Job drawing, mm, ordinate dimensions from the low corner. One solid piece. A direction names the side the tool comes from. Coordinates: 2 decimals unless noted, no trailing zeros. Loops run counter-clockwise (first coordinate to the right, second up) from the corner with the lowest first, then second, coordinate; pieces in that order, holes last. Notation, with made-up numbers: (14, -3.75) -> (71, -3.75) arc R11 cw to (71, 13.25) -> close; hole circle Ø3 at (42.5, 49). An arc over 180 degrees is marked (long way). Answer as CSV lines item,"result". Start each with the question number.
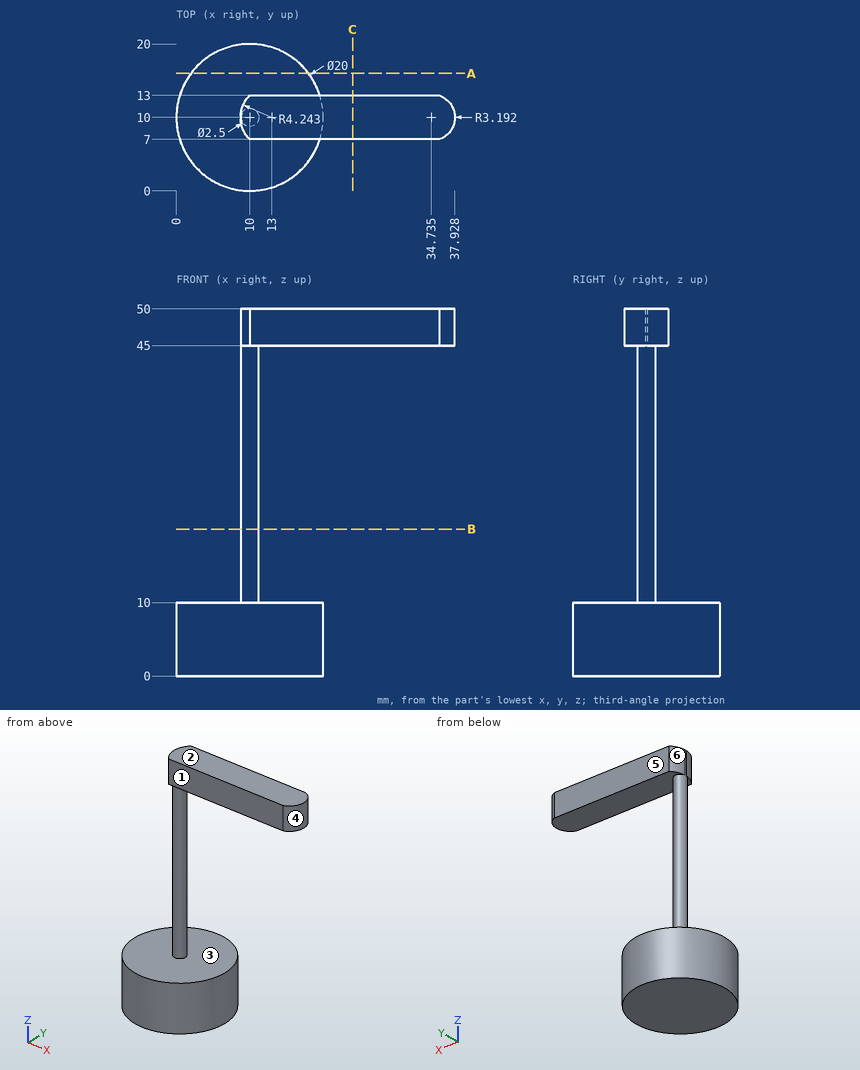
Item 1: Flat gauge pins, fed straight in: pin 1 Ø4 at (x, z) = (28, 48.5) entering from -Y; pin 2 Ø8 at (y, z) = (15, 28) entering from +X; pin 3 Ø10 at (x, y) = (31.5, 10) entering from -Z. Where does each tip first touch, or does it go through?
Item 2: Wall check: probe 1 along Z at (x, y) = (18, 8); probe 2 along Z at (x, y) = (33, 11.75); probe 3 along Y at (x, z) = (10, 32). Give the ranges that are in metal, low to high.
Item 3: Two-plate mould, pull along Z, no slides. Class the marked faces 1, 2 and 3: pulls with the +Z half, pulls with the -Z half, needs draft (parallel to the pull), parting line crosses it, or undercut.
Item 4: Saw through at B-B (z = 20). Write the cut outline in (x, y).
Item 5: Saw through at C-C (x = 24). Write the cut outline in (y, z).
Item 6: Which spindle directions (+Z, -Z, +X, -X, +Y, -Y) get a long thin tool onto all of the face, cutting with end or side? Do the marked faces 4, 5 and 6. Say none if no direction does.
Item 7: Saw through at A-A (y = 16). Write the cut outline in (x, z), plus the area to 3 significant figures.
Geometry check:
1,pin 1,"y = 7"
1,pin 2,"x = 10.75"
1,pin 3,"z = 45"
2,probe 1,"0 to 10, 45 to 50"
2,probe 2,"45 to 50"
2,probe 3,"8.75 to 11.25"
3,face 1,"needs draft"
3,face 2,"pulls with the +Z half"
3,face 3,"undercut"
4,outline,"circle Ø2.5 at (10, 10)"
5,outline,"(7, 45) -> (13, 45) -> (13, 50) -> (7, 50) -> close"
6,face 4,"+Z, -Z, +X"
6,face 5,"+Z, +X, -X, +Y"
6,face 6,"+Z, -X, +Y"
7,outline,"(2, 0) -> (18, 0) -> (18, 10) -> (2, 10) -> close"
7,area,"160 mm2"
